Part model, mm, in its own coordinate system. A direction names the side the tool comes from. Coordinates: 2 decimals unless noted, no trailing zeros. Order: outer loops, then holes, each group sorted by start corner. A loop starts at its lowest first (then second) coordinate and runs counter-clockwise, first axis right, second up.
1) Cut at A-A (z = 0). List the corners of the cut face in (x, y), and give its area (3 significant figures).
2) Tool access for faces 1 (the flat face through (-1.24, -0.99, 2.17)), 2 (the flat face through (0, -34, 0)), 3 (the flat face through (2, -4, 2)): list every direction of +Z, -Z, +X, -X, +Y, -Y with a clear straight run to the whole face (end or side of a thin tool).
3) Mould opens along Z. For faces 4 (the flat face through (0, -2, 0)), 5 (the cylindrical face through (3.233, -1.972, 1.341)), 6 (the flat face through (1.24, -0.99, -2.17)), 7 (the flat face through (3, 0, 0)) say: +Z half, -Z half, draft (parallel to the pull), parting line (faces both ways), or undercut.
4) Cut at B-B (y = -30.5). List the corners of the cut face in (x, z), and give its area (3 significant figures).
5) Wall check: L1, parallel to Y at x = -2, z = 0.5; L2, parallel to Y at x = -1, z = 3; L3, parallel to X at y = -1.5, z = -2.75. Give the ranges that are in metal, low to high.
6) Pin check, flat tips, straight feed: pin 1 Ø1.5 at (x, y) = (-2, -12.5) entering from +Z; pin 2 Ø1.5 at (y, z) = (-24, 2) entering from -X; pin 3 Ø1.5 at (x, y) = (-2.5, -15) entering from -Z. Stop position of each tip, or through.
```python
from build123d import *

# Parameters (mm, degrees)
SKETCH_1_R          = 3.5
EXTRUDE_1_DEPTH     = 4
SKETCH_2_R          = 2
EXTRUDE_2_DEPTH     = 30
CUT_EXTRUDE_1_DEPTH = 2


with BuildPart() as part:
    # 草图1 → 凸台-拉伸1 (new body)
    with BuildSketch(Plane(origin=(0, 0, 0), x_dir=(1, 0, 0), z_dir=(0, 1, 0))):
        Circle(SKETCH_1_R)
    extrude(amount=-EXTRUDE_1_DEPTH)

    # 草图2 → 凸台-拉伸2 (add)
    with BuildSketch(Plane.XZ.offset(4)):
        Circle(SKETCH_2_R)
    extrude(amount=EXTRUDE_2_DEPTH)

    # 草图3 → 切除-拉伸1 (cut)
    with BuildSketch(Plane(origin=(0, 0, 0), x_dir=(1, 0, 0), z_dir=(0, 1, 0))):
        Polygon((2.51555192, -1.416097409), (2.484152291, 1.470483162), (-0.031399629, 2.886580572), (-2.51555192, 1.416097409), (-2.484152291, -1.470483162), (0.031399629, -2.886580572), align=None)
    extrude(amount=-CUT_EXTRUDE_1_DEPTH, mode=Mode.SUBTRACT)


solid = part.part
```
Geometry check:
1. outline: (-3.5, -4) - (-2, -4) - (-2, -34) - (2, -34) - (2, -4) - (3.5, -4) - (3.5, 0) - (2.5, 0) - (2.5, -2) - (-2.5, -2) - (-2.5, 0) - (-3.5, 0) - close
1. area: 138 mm2
2. face 1: +Y
2. face 2: +Z, -Z, +X, -X, -Y
2. face 3: -Y
3. face 4: undercut
3. face 5: parting line
3. face 6: undercut
3. face 7: draft
4. outline: circle Ø4 at (0, 0)
4. area: 12.6 mm2
5. L1: y = -4 to -2
5. L2: y = -4 to 0
5. L3: x = -2.17 to -0.26, 0.21 to 2.17
6. pin 1: stops at z = 1.56
6. pin 2: stops at x = -1.56
6. pin 3: stops at z = -0.97
